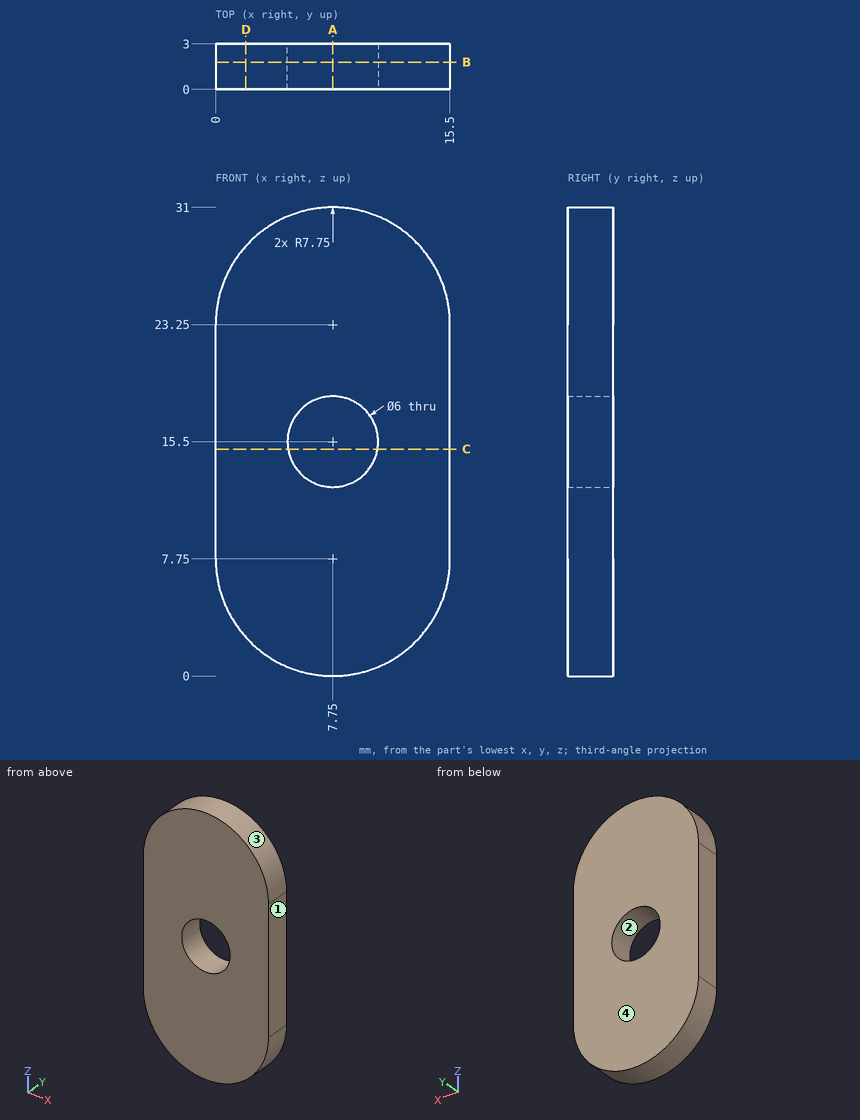
Input: dimensioned drawing with shaded views. Units: mm. Origin: part minimum x, y, z. Give positions to 0.01 mm unless a question says otherwise; leave off trailing zeros. Write each loop counter-clockwise with the first axis right and the second up, starting at its lowest first coordinate (ties: lowest second). Pieces come first, ordered by that corner, then holes.
1. Section query A-A (x = 7.75). Return the cut outline in (y, z).
2. First-contact query: pin 1 (1 mm diameter, centred on x = 14, y = 2.5, fed in from -Z); pin 2 (1.5 mm diameter, centred on x = 12.5, y = 0.5, fed in from -Z). Flat tips, straight axial feed; report the tip coordinate or a pass-through.
3. Section query D-D (x = 2). Return the cut outline in (y, z), then the cut area to 3 significant figures.
4. Pull-direction query (X, two-part tool) for the marked faces 1, 2, 3 and 4; classes: +X half, -X half, draft (parallel to the pull), parting line (faces both ways), or undercut.
5. Section query B-B (y = 1.8). Return the cut outline in (x, z), then the cut area to 3 significant figures.
6. Material intervals for line 1 along Z through (x, y) = (7.75, 0.8); line 2 along X through (y, z) = (2.5, 23.5); line 3 along X through (y, z) = (0.2, 15), sorted ascending.
7. Section query C-C (z = 15). Return the cut outline in (x, y).
Output values:
1. outline: (0, 0) - (3, 0) - (3, 12.5) - (0, 12.5) - close; (0, 18.5) - (3, 18.5) - (3, 31) - (0, 31) - close
2. pin 1: stops at z = 2.55
2. pin 2: stops at z = 1.11
3. outline: (0, 2.55) - (3, 2.55) - (3, 28.45) - (0, 28.45) - close
3. area: 77.7 mm2
4. face 1: +X half
4. face 2: undercut
4. face 3: parting line
4. face 4: draft
5. outline: (0, 7.75) arc R7.75 ccw to (15.5, 7.75) - (15.5, 23.25) arc R7.75 ccw to (0, 23.25) - close; hole circle Ø6 at (7.75, 15.5)
5. area: 401 mm2
6. line 1: z = 0 to 12.5, 18.5 to 31
6. line 2: x = 0 to 15.5
6. line 3: x = 0 to 4.79, 10.71 to 15.5
7. outline: (0, 0) - (4.79, 0) - (4.79, 3) - (0, 3) - close; (10.71, 0) - (15.5, 0) - (15.5, 3) - (10.71, 3) - close
